Read the model definition and answer for the solid it produces. Units are mm, in the model's axes. A direction names the side the tool comes from. Coordinates: 2 decimals unless noted, no trailing zeros. Loops run counter-clockwise (first coordinate to the right, second up) from the corner with the lowest first, then second, coordinate; pieces in that order, holes last. Notation, with made-up numbers: M 46.5,-11 L 62.5,-11 A4 cw 62.5,-6 Z; hole C 29,-11 d9. An arc over 180 degrees is marked long. One line per item, written item: value. Start each with the question number.
1. For faces 1 (the face through (5.426, -14.628, 6.93)), 2 (the face through (67.096, -14.55, 6.93)), 3 (the face through (36, -13.125, 7)), 4 (the face through (5.504, -21.7, 6.93)), 5 (the face through (67.174, -21.622, 6.93)), determine the directions among +Z, -Z, +X, -X, +Y, -Y from which every point of the face is accessible in a straight line to the end or side of a thin tool.
2. Determine the mould class of faces 6 (the face through (37, -23.125, 7)), 7 (the face through (8.827, -20.004, 6.084)), 8 (the face through (19.127, -20.004, 6.084)), 9 (the face through (0, -18, 1)) for opening direction X: +X half, -X half, draft (parallel to the pull), parting line (faces both ways), or undercut.
3. Consider probe 1 along Z at (x, y) = (51, -10.5); probe 2 along Y at (x, z) = (37, 5.5) (3 decimals); probe 3 along Y at (x, z) = (41, 10) (3 decimals). Determine where each line is inside the solid, lowest interval first.
4. The part is cut by section B-B (z = 10.5). Write down the section's boundary in (x, y) (3 decimals), then the cut area to 3 significant figures.
5. The part is cut by section D-D (x = 51). Write down the section's boundary in (y, z) (3 decimals).
6. The part is cut by section C-C (x = 27). Write down the section's boundary in (y, z) (3 decimals), then the cut area to 3 significant figures.
7. Flat-ended cylindrical pins translate along their axes: pin 1 (2 mm diameter, centred on x = 58, z = 5.5, fed in from -Y) (3 decimals); pin 2 (2 mm diameter, centred on x = 33.5, z = 4, fed in from +Y) (3 decimals); pin 3 (5 mm diameter, centred on y = -22.5, z = 6, fed in from -X). Find the tip coordinate at first contact, or state that the pin passes through.
8. The part is cut by section A-A (x = 62.05). Write down the section's boundary in (y, z) (3 decimals).
Autodesk Fusion 360 part; units mm, degrees
sketch "スケッチ1" plane through (0, 0, 0) normal (0, 0, 1) x (1, 0, 0)
  line L0 (0, 0) -> (72.6, 0)
  line L1 (72.6, 0) -> (72.6, -36.25)
  line L2 (72.6, -36.25) -> (0, -36.25)
  line L3 (0, -36.25) -> (0, 0)
  line L4 (36.3, 0) -> (36.3, -36.25)
  line L5 (0, -18.125) -> (72.6, -18.125)
  line L6 (72.6, -8.625) -> (72.6, -26.625)
  line L7 (58.3, -36.25) -> (14.3, -36.25)
  line L8 (0, -9.125) -> (0, -27.125)
  line L9 (0, -18.125) -> (9.5, -18.125)
  line L10 (0, -9.125) -> (6.4586, -9.125)
  line L11 (0, -27.125) -> (4.6488, -27.125)
  line L12 (6.4586, -9.125) -> (36.3, 0)
  line L13 (14.3, -36.25) -> (12.3, -36.25)
  line L14 (12.3, -36.25) -> (2.2204, -24.2289)
  line L15 (36.3, -18.125) -> (36.3, -32.425)
  line L16 (36.3, -18.125) -> (36.3, -3.825)
  line L17 (66.1414, -9.125) -> (36.3, 0)
  line L18 (60.3, -36.25) -> (70.3796, -24.2289)
  line L19 (58.3, -36.25) -> (60.3, -36.25)
  line L20 (6.4586, -27.125) -> (66.1414, -27.125)
  line L21 (6.4586, -9.125) -> (66.1414, -9.125)
  arc A0 (6.9878, -8.9632) -> (6.4586, -27.125) centre (9.5, -18.125) ccw
  arc A1 (66.1414, -27.125) -> (65.6122, -8.9632) centre (63.1, -18.125) ccw
  circle A2 centre (14.3, -32.425) radius 1.75
  circle A3 centre (36.3, -3.825) radius 1.75
  circle A4 centre (58.3, -32.425) radius 1.75
  circle A5 centre (32.3, -32.425) radius 1
  circle A6 centre (40.3, -32.425) radius 1
  point P0 (36.3, -18.125)
  point P1 (36.3, -3.825)
  point P2 (14.3, -32.425)
  point P3 (58.3, -32.425)
  point P4 (40.3, -32.425)
  point P5 (40.3, -32.425)
  point P6 (32.3, -32.425)
  dimension "d5" = 72.6
  dimension "d6" = 36.25
  dimension "d10" = 44
  dimension "d11" = 9
  dimension "d12" = 18
  dimension "d13" = 9.5
  dimension "d14" = 2
  dimension "d15" = 14.3
  dimension "d16" = 22
  dimension "d17" = 14.3
  dimension "d18" = 3.5
  dimension "d19" = 3.5
  dimension "d20" = 3.5
  dimension "d21" = 4
  dimension "d24" = 2
  dimension "d25" = 2
extrude "押し出し2" add sketch "スケッチ1" along normal blind 12 contours L4 L5 L9 L16 L21 A0 | L4 L5 L9 L15 L20 A0 | L4 L5 L16 L21 A1 | L4 L5 L15 L20 A1
sketch "スケッチ3" plane through (0, 0, 0) normal (0, 0, -1) x (1, 0, 0)
  arc A0 (6.4586, 27.125) -> (6.4586, 9.125) centre (9.5, 18.125) ccw
  line L0 (6.4586, 9.125) -> (66.1414, 9.125)
  arc A1 (66.1414, 9.125) -> (66.1414, 27.125) centre (63.1, 18.125) ccw
  line L1 (66.1414, 27.125) -> (6.4586, 27.125)
  line L2 (72.6, 18.125) -> (0, 18.125)
  line L3 (72.6, 18.125) -> (36.3, 18.125)
  line L4 (36.3, 18.125) -> (31.15, 18.125)
  line L5 (31.15, 18.125) -> (20.85, 18.125)
  line L6 (20.85, 18.125) -> (10.55, 18.125)
  line L7 (36.3, 18.125) -> (36.3, 27.125)
  point P0 (36.3, 18.125)
  point P1 (31.15, 18.125)
  point P2 (20.85, 18.125)
  point P3 (10.55, 18.125)
  point P4 (41.45, 18.125)
  point P5 (51.75, 18.125)
  point P6 (62.05, 18.125)
  dimension "d32" = 5.15
  dimension "d33" = 10.3
  dimension "d34" = 10.3
hole "穴1" at (62.05, -18.125, 0) at (51.75, -18.125, 0) at (41.45, -18.125, 0) at (31.15, -18.125, 0) at (20.85, -18.125, 0) at (10.55, -18.125, 0) direction (0, 0, 1) diameter 5.1 depth 12 tip angle 180
sketch "スケッチ4" plane through (0, 0, 12) normal (0, 0, 1) x (-1, 0, 0)
  circle A0 centre (-20.85, 18.125) radius 2.55
  circle A1 centre (-41.45, 18.125) radius 2.55
  circle A2 centre (-62.05, 18.125) radius 2.55
  circle A3 centre (-51.75, 18.125) radius 2.55
  circle A4 centre (-31.15, 18.125) radius 2.55
  circle A5 centre (-10.55, 18.125) radius 2.55
  arc A6 (-6.4586, 9.125) -> (-6.4586, 27.125) centre (-9.5, 18.125) ccw
  line L0 (-6.4586, 27.125) -> (-66.1414, 27.125)
  arc A7 (-66.1414, 27.125) -> (-66.1414, 9.125) centre (-63.1, 18.125) ccw
  line L1 (-66.1414, 9.125) -> (-6.4586, 9.125)
  line L2 (0, 18.125) -> (-4, 18.125)
  line L3 (-36.3, 13.125) -> (-5.4223, 13.125)
  line L4 (-4, 18.125) -> (-13.5, 18.125)
  line L5 (-36.3, 23.125) -> (-5.4223, 23.125)
  line L6 (-36.3, 23.125) -> (-36.3, 27.125)
  arc A8 (-5.4223, 13.125) -> (-5.4223, 23.125) centre (-13.5, 18.125) ccw
  line L7 (-36.3, 13.125) -> (-67.1777, 13.125)
  arc A9 (-67.1777, 23.125) -> (-67.1777, 13.125) centre (-59.1, 18.125) ccw
  line L8 (-36.3, 23.125) -> (-67.1777, 23.125)
  line L9 (-36.3, 23.125) -> (-36.3, 13.125)
  line L10 (-31.15, 18.125) -> (-41.45, 18.125)
  point P0 (-68.6, 18.125)
  dimension "d39" = 9.5
  dimension "d40" = 4
  dimension "d45" = 4
  dimension "d46" = 5.1
  dimension "d47" = 9.5
  dimension "d48" = 10.3
extrude "押し出し3" cut sketch "スケッチ4" against normal blind 10 contours A6 L0 L2 L5 L6 A8 | A6 L0 A7 L1 L2 L3 L6 A8 L7 A9 L8
fillet "フィレット2" radius 5 4 edges at (5.4223, -23.125, 7) (5.4223, -13.125, 7) (67.1777, -13.125, 7) (67.1777, -23.125, 7)
Answer block:
1. face 1: +Z, -X, +Y
1. face 2: +Z, +X, +Y
1. face 3: +Z, +X, -X, +Y
1. face 4: +Z, -X, -Y
1. face 5: +Z, +X, -Y
2. face 6: draft
2. face 7: undercut
2. face 8: undercut
2. face 9: -X half
3. probe 1: z = 0 to 2
3. probe 2: y = -23.125 to -13.125
3. probe 3: y = -23.125 to -20.635, -15.615 to -13.125
4. outline: M 4,-18.127 A4.999 ccw 8.999,-23.125 L 63.601,-23.125 A4.999 ccw 68.6,-18.127 A9.5 ccw 68.6,-18.123 A4.999 ccw 63.601,-13.125 L 8.999,-13.125 A4.999 ccw 4,-18.123 A9.5 ccw Z; hole C 10.55,-18.125 d5.1; hole C 20.85,-18.125 d5.1; hole C 31.15,-18.125 d5.1; hole C 41.45,-18.125 d5.1; hole C 51.75,-18.125 d5.1; hole C 62.05,-18.125 d5.1
4. area: 502 mm2
5. outline: M -27.125,0 L -20.562,0 L -20.562,12 L -23.125,12 L -23.125,2 L -27.125,2 Z; M -15.688,0 L -9.125,0 L -9.125,2 L -13.125,2 L -13.125,12 L -15.688,12 Z
6. outline: M -27.125,0 L -9.125,0 L -9.125,2 L -13.125,2 L -13.125,12 L -23.125,12 L -23.125,2 L -27.125,2 Z
6. area: 136 mm2
7. pin 1: stops at y = -23.125
7. pin 2: stops at y = -13.125
7. pin 3: stops at x = 4.36
8. outline: M -27.125,0 L -20.675,0 L -20.675,12 L -23.125,12 L -23.125,2 L -27.125,2 Z; M -15.575,0 L -9.125,0 L -9.125,2 L -13.125,2 L -13.125,12 L -15.575,12 Z
